Source: CAD feature listing. Evaluate the final solid. Frame: model axes, mm. A direction names the side the tool comes from. Coordinates: 2 decimals unless noted, no trailing zeros. Order: outer loops, then holes, each group sorted by start corner. A loop starts at its lowest first (then second) coordinate and runs counter-clockwise, first axis right, second up. Notation, with made-up numbers: (18, 79.5) - (50, 79.5) arc R21 cw to (50, 86.5) - close; hole circle Ø8 at (85, -0.75). An arc over 180 degrees is marked (long way). One line per question, with ' | ' between items.
from build123d import *

# Parameters (mm, degrees)
SKETCH1_R           = 3.55
SKETCH1_R_2         = 1.5
BOSS_EXTRUDE1_DEPTH = 6
SKETCH2_W           = 6
SKETCH2_H           = 20
CUT_EXTRUDE1_DEPTH  = 1


with BuildPart() as part:
    # Sketch1 → Boss-Extrude1 (new body)
    with BuildSketch(Plane(origin=(0, 0, 0), x_dir=(0, 0, -1), z_dir=(1, 0, 0))):
        with BuildLine():
            Line((-7, 10), (-1.033439229, 11.843950263))
            ThreePointArc((-1.033439229, 11.843950263), (0.525907674, 11.960263157), (1.980283773, 11.38590994))
            Line((1.980283773, 11.38590994), (4, 10))
            Line((4, 10), (4, -10))
            Line((4, -10), (1.980283773, -11.38590994))
            ThreePointArc((1.980283773, -11.38590994), (0.525907674, -11.960263157), (-1.033439229, -11.843950263))
            Line((-1.033439229, -11.843950263), (-7, -10))
            Line((-7, -10), (-19, -10))
            Line((-19, -10), (-19, 10))
            Line((-19, 10), (-7, 10))
        make_face()
        Circle(SKETCH1_R, mode=Mode.SUBTRACT)
        with Locations((0, -8.5)):
            Circle(SKETCH1_R_2, mode=Mode.SUBTRACT)
        with Locations((0, 8.5)):
            Circle(SKETCH1_R_2, mode=Mode.SUBTRACT)
    extrude(amount=BOSS_EXTRUDE1_DEPTH)

    # Sketch2 → Cut-Extrude1 (cut)
    with BuildSketch(Plane.ZY):
        with Locations((10, 0)):
            Rectangle(SKETCH2_W, SKETCH2_H)
    extrude(amount=-CUT_EXTRUDE1_DEPTH, mode=Mode.SUBTRACT)


solid = part.part
(1) Cut plane C-C (x = 1.7). Return the cut outline in (y, z).
Taken from the geometry:
outline: (-11.84, 1.03) arc R3.5 ccw to (-11.39, -1.98) - (-10, -4) - (10, -4) - (11.39, -1.98) arc R3.5 ccw to (11.84, 1.03) - (10, 7) - (10, 19) - (-10, 19) - (-10, 7) - close; hole circle Ø3 at (-8.5, 0); hole circle Ø7.1 at (0, 0); hole circle Ø3 at (8.5, 0)
(2) Cut plane D-D (z = 2.75). Return the cut outline in (x, y) (3 decimals), and give its area (3 significant figures).
Taken from the geometry:
outline: (0, -11.313) - (6, -11.313) - (6, -2.245) - (0, -2.245) - close; (0, 2.245) - (6, 2.245) - (6, 11.313) - (0, 11.313) - close | area: 109 mm²
(3) Material intervals for L1, parallel to Y at x = 4.85, z = 0; L2, parallel to Z at x = 0.4, y = 1; L3, parallel to X at y = -6.75, z = 9.5, sorted ascending. Write a range as from..to.
Taken from the geometry:
L1: y = -12..-10, -7..-3.55, 3.55..7, 10..12 | L2: z = -4..-3.41, 3.41..7, 13..19 | L3: x = 1..6
(4) Set-up query: faces 4 (the flat face through (6, 0, 7)), 5 (the flat face through (3, 10, 13)), 6 (the flat face through (3, -10, 13)), 7 (the flat face through (1, 0, 10)). Return all of +Z, -Z, +X, -X, +Y, -Y with unobstructed straight access to the full face (end or side cutting, diameter ignored); none if empty.
Taken from the geometry:
face 4: +Z, -Z, +X, +Y, -Y | face 5: +Z, +X, -X, +Y | face 6: +Z, +X, -X, -Y | face 7: -X, +Y, -Y
(5) Cut plane A-A (y = 8.5). Return the cut outline in (x, z), and give its area (3 significant figures).
Taken from the geometry:
outline: (0, -4) - (6, -4) - (6, -1.5) - (0, -1.5) - close; (0, 1.5) - (6, 1.5) - (6, 19) - (0, 19) - (0, 13) - (1, 13) - (1, 7) - (0, 7) - close | area: 114 mm²
(6) Cut plane B-B (z = 0). Return the cut outline in (x, y).
Taken from the geometry:
outline: (0, -12) - (6, -12) - (6, -10) - (0, -10) - close; (0, -7) - (6, -7) - (6, -3.55) - (0, -3.55) - close; (0, 3.55) - (6, 3.55) - (6, 7) - (0, 7) - close; (0, 10) - (6, 10) - (6, 12) - (0, 12) - close
(7) Pin query (flat end, axial travel): P1, Ø3, axis at x = 2, z = 9.5, coming from the +Y side; P2, Ø1.5, axis at x = 2.5, z = 12, coming from the -Y side; P3, Ø5.5, axis at y = 0, z = 0, coming from the +X side. Return the tip coordinate at first contact, or that it passes through.
Taken from the geometry:
P1: stops at y = 10 | P2: stops at y = -10 | P3: passes through
(8) Pull-direction query (Z, two-part tool) for faces 1 (the flat face through (2.958, -10.683, -3.004)), 2 (the cylindrical face through (2.96, 3.52, 0.46)), 3 (the flat face through (3, 0, 19)); classes: pulls with the +Z half, pulls with the -Z half, needs draft (parallel to the pull), parting line crosses it, or undercut.
Taken from the geometry:
face 1: pulls with the -Z half | face 2: undercut | face 3: pulls with the +Z half
